Geometry: final body of the model. Coordinates: model frame, mm. A direction names the side the tool comes from. Round coordinates to 2 decimals unless told otherwise and drop trailing zeros. Order: outer loops, then holes, each group sorted by start corner. A loop starts at its lowest first (then second) coordinate and runs counter-clockwise, first axis right, second up. Notation, with made-up numbers: (-39.5, 45.25) -> (-29.5, 45.25) arc R21 ccw to (-29.5, 54.25) -> close; hole circle Ø6 at (43.5, -5.5). An arc over 180 degrees is marked (long way). Put each result on its own line as item: value.
```python
from build123d import *

# Parameters (mm, degrees)
F0_W          = 6.35
F0_H          = 28.448
F1_DEPTH      = 14.224
F3_W          = 4.826
F3_H          = 10.922
F4_DEPTH      = 73.407
F4_DEPTH_BACK = 31.243
F2_W          = 3.81
F2_H          = 1.524
F2_W_2        = 6.35
F2_H_2        = 4.826
F5_DEPTH      = 28.448


with BuildPart() as f1:
    # F0 (on Front) → F1 (new body, symmetric)
    with BuildSketch(Plane.XZ):
        Polygon((0, 0), (0, 14.2875), (-67.056, 14.2875), (-73.406, 14.2875), (-73.406, 0), align=None)
        Polygon((-67.056, 14.2875), (0, 14.2875), (2.794, 14.2875), (13.716, 25.2095), (-3.5814, 25.2095), (-3.5814, 42.7355), (-67.056, 42.7355), align=None)
        with BuildLine():
            Line((-19.304, 22.9235), (-43.18, 22.9235))
            ThreePointArc((-43.18, 22.9235), (-48.768, 28.5115), (-43.18, 34.0995))
            Line((-43.18, 34.0995), (-19.304, 34.0995))
            ThreePointArc((-19.304, 34.0995), (-13.716, 28.5115), (-19.304, 22.9235))
        make_face(mode=Mode.SUBTRACT)
        with Locations((-70.231, 28.5115)):
            Rectangle(F0_W, F0_H)
        Polygon((-3.5814, 25.2095), (13.716, 25.2095), (31.242, 42.7355), (-3.5814, 42.7355), align=None)
    extrude(amount=F1_DEPTH, both=True)

    # F3 (on face) → F4 (cut, two sides)
    with BuildSketch(Plane.YZ) as f4_sk:
        Polygon((-14.224, 42.7355), (-14.224, 14.2875), (-12.7, 14.2875), (-12.7, 25.2095), (-12.7, 42.7355), align=None)
        with Locations((-10.287, 19.7485)):
            Rectangle(F3_W, F3_H)
        Polygon((12.7, 14.2875), (14.224, 14.2875), (14.224, 42.7355), (12.7, 42.7355), (12.7, 25.2095), align=None)
        with Locations((10.287, 19.7485)):
            Rectangle(F3_W, F3_H)
    extrude(amount=-F4_DEPTH, mode=Mode.SUBTRACT)
    extrude(f4_sk.sketch, amount=F4_DEPTH_BACK, mode=Mode.SUBTRACT)

    # F2 (on face) → F5 (cut, through all)
    with BuildSketch(Plane.XY.offset(42.7355)):
        Polygon((-3.81, 14.224), (-73.406, 14.224), (-73.406, 7.874), (-3.81, 7.874), (-3.81, 12.7), align=None)
        with Locations((-1.905, 13.462)):
            Rectangle(F2_W, F2_H)
        with Locations((-1.905, -13.462)):
            Rectangle(F2_W, F2_H)
        Polygon((-73.406, -14.224), (-3.81, -14.224), (-3.81, -12.7), (-3.81, -7.874), (-67.056, -7.874), (-73.406, -7.874), align=None)
        with Locations((-70.231, -5.461)):
            Rectangle(F2_W_2, F2_H_2)
    extrude(amount=-F5_DEPTH, mode=Mode.SUBTRACT)

    # F6: F1 across plane


with BuildPart() as f1_1:
    add(f1.part)
    add(f1.part.mirror(Plane.XY))


solid = f1_1.part
```
1. Set-up query: faces 5 (the face through (1, 0, 14.288)), 6 (the face through (-48.767, -0.11, 28.389)), 7 (the face through (-3.81, 10, -34)), 8 (the face through (10, -12.7, -34)), 9 (the face through (5, 10, -25.21)). Return all of +Z, -Z, +X, -X, +Y, -Y with unobstructed straight access to the full face (end or side cutting, diameter ignored); none if empty.
Ans:
face 5: +X, +Y, -Y
face 6: +Y, -Y
face 7: -Z, -X, +Y
face 8: -Z, +X, -X, -Y
face 9: +X, -X, +Y
2. Draft query along Z for faces 1 (the face through (-31, 0, -22.924)), 2 (the face through (-37, -14.224, 0)), 3 (the face through (-13.717, -0.11, 28.634)), 4 (the face through (-9, 0, -42.736)). Return one class per face: +Z half, -Z half, draft (parallel to the pull), parting line (faces both ways), or undercut.
Ans:
face 1: undercut
face 2: draft
face 3: undercut
face 4: -Z half
3. Cut plane A-A on x = -22. Return loops of the section in (y, z).
Ans:
outline: (-14.22, -14.29) -> (-7.87, -14.29) -> (-7.87, -22.92) -> (7.87, -22.92) -> (7.87, -14.29) -> (14.22, -14.29) -> (14.22, 14.29) -> (7.87, 14.29) -> (7.87, 22.92) -> (-7.87, 22.92) -> (-7.87, 14.29) -> (-14.22, 14.29) -> close; (-7.87, -42.74) -> (7.87, -42.74) -> (7.87, -34.1) -> (-7.87, -34.1) -> close; (-7.87, 34.1) -> (7.87, 34.1) -> (7.87, 42.74) -> (-7.87, 42.74) -> close
4. Cut plane B-B on y = -9.5. Return loops of the section in (x, z).
Ans:
outline: (-73.41, -14.29) -> (0, -14.29) -> (0, 14.29) -> (-73.41, 14.29) -> close; (-3.81, -42.74) -> (31.24, -42.74) -> (13.72, -25.21) -> (-3.81, -25.21) -> close; (-3.81, 25.21) -> (13.72, 25.21) -> (31.24, 42.74) -> (-3.81, 42.74) -> close
5. Contact query for flat-ended pins moving along their axis: P1, Ø1.5, axis at x = -41, y = 11.5, coming from the -Z side; P2, Ø1.9, axis at x = -34, y = 11, coming from the +Z side; P3, Ø4, axis at y = -6, z = 29.5, coming from the -X side. Output: stop coordinate, or through.
Ans:
P1: z = -14.29
P2: z = 14.29
P3: x = -67.06
6. Material intervals for probe 1 along Z at (x, y) = (-3, -12.5); probe 2 along Z at (x, y) = (0.5, 12.25); probe 3 along Z at (x, y) = (-57.5, -11), sorted ascending.
Ans:
probe 1: -42.74 to -25.21, -14.29 to 14.29, 25.21 to 42.74
probe 2: -42.74 to -25.21, 25.21 to 42.74
probe 3: -14.29 to 14.29
7. Cut plane C-C on z = 30. Return loops of the section in (x, y), and give its area (3 significant figures).
Ans:
outline: (-73.41, -3.05) -> (-67.06, -3.05) -> (-67.06, -7.87) -> (-48.57, -7.87) -> (-48.57, 7.87) -> (-73.41, 7.87) -> close; (-13.92, -7.87) -> (-3.81, -7.87) -> (-3.81, -12.7) -> (18.51, -12.7) -> (18.51, 12.7) -> (-3.81, 12.7) -> (-3.81, 7.87) -> (-13.92, 7.87) -> close
area: 1,090 mm²
8. Cut plane D-D on x = -11.5. Return loops of the section in (y, z), and give its area (3 significant figures).
Ans:
outline: (-14.22, -14.29) -> (-7.87, -14.29) -> (-7.87, -42.74) -> (7.87, -42.74) -> (7.87, -14.29) -> (14.22, -14.29) -> (14.22, 14.29) -> (7.87, 14.29) -> (7.87, 42.74) -> (-7.87, 42.74) -> (-7.87, 14.29) -> (-14.22, 14.29) -> close
area: 1,710 mm²
